Input: part model. Units: mm. Frame: model coordinates. Coordinates: 2 decimals unless noted, no trailing zeros. Write each loop counter-clockwise with the first axis right and the second up, starting at its lowest first coordinate (ties: lowest second). Pieces come first, ordered by that corner, then holes. Notation, with made-up numbers: M 0.5,21 L 38.5,21 A26 ccw 38.5,47 Z; hole C -30,-14.5 d9. An arc over 180 degrees is marked long. Use CSV: the item, a comma, the result in double quotes.
```python
from build123d import *

# Parameters (mm, degrees)
F0_R     = 2.5
F1_DEPTH = 5


with BuildPart() as f1:
    # F0 (on Top) → F1 (new body)
    with BuildSketch(Plane.XY):
        with BuildLine():
            Line((-16, -5), (0, -5))
            ThreePointArc((0, -5), (3.535534, -3.535534), (5, 0))
            Line((5, 0), (5, 15))
            ThreePointArc((5, 15), (0, 20), (-5, 15))
            ThreePointArc((-5, 15), (-8.273146, 7.550461), (-16, 5))
            ThreePointArc((-16, 5), (-21, 0), (-16, -5))
        make_face()
        with Locations((-16, 0)):
            Circle(F0_R, mode=Mode.SUBTRACT)
        with Locations((0, 15)):
            Circle(F0_R, mode=Mode.SUBTRACT)
    extrude(amount=F1_DEPTH)


solid = f1.part
```
1. Section A-A (z = 1.15). Return loops of the section in (x, y), then the cut area to 3 significant figures.
Resolved:
outline,"M -16,-5 L 0,-5 A5 ccw 5,0 L 5,15 A5 ccw -5,15 A10 cw -16,5 A5 ccw Z; hole C -16,0 d5; hole C 0,15 d5"
area,"365 mm^2"
2. Section B-B (x = -14.5). Return loops of the section in (y, z), then the cut area to 3 significant figures.
Resolved:
outline,"M -5,0 L -2,0 L -2,5 L -5,5 Z; M 2,0 L 4.96,0 L 4.96,5 L 2,5 Z"
area,"29.8 mm^2"
3. Mould query, pull axis Y, two halves, no side actions, for faces 1 (the flat face through (-8, -5, 2)), 2 (the cylindrical face through (-18.5, 0.1, 2.5)), 3 (the cylindrical face through (-0.54, 12.56, 2.46)), 4 (the flat face through (-5, 5, 0)). Classes: pulls with the +Y half, pulls with the -Y half, needs draft (parallel to the pull), parting line crosses it, or undercut.
Resolved:
face 1,"pulls with the -Y half"
face 2,"undercut"
face 3,"undercut"
face 4,"needs draft"
4. Material intervals for line 1 (Y direction, x = 0, z = 1.3); line 2 (Y direction, x = -16, z = 2.3); line 3 (X direction, y = 17, z = 1.9), sorted ascending. Write a range as [from, to].
Resolved:
line 1,"y = [-5, 12.5], [17.5, 20]"
line 2,"y = [-5, -2.5], [2.5, 5]"
line 3,"x = [-4.58, -1.5], [1.5, 4.58]"
5. Section D-D (x = -9.5). Return loops of the section in (y, z).
Resolved:
outline,"M -5,0 L 6.6,0 L 6.6,5 L -5,5 Z"
6. Section C-C (y = -1.5). Return loops of the section in (x, z).
Resolved:
outline,"M -20.77,0 L -18,0 L -18,5 L -20.77,5 Z; M -14,0 L 4.77,0 L 4.77,5 L -14,5 Z"
7. Contact query for a flat-ended pin moving along its axis: pin 1 Ø3 at (x, y) = (-16, 0) entering from -Z. Output: stop coordinate, or through.
Resolved:
pin 1,"passes through"
